```python
from build123d import *

# Parameters (mm, degrees)
F1_DEPTH = 346.075
F3_DEPTH = 31.751
F5_DEPTH = 38.1


with BuildPart() as f1:
    # F0 (on Front) → F1 (new body)
    with BuildSketch(Plane.XZ):
        with BuildLine():
            Line((0, -25.4), (0, 0))
            Line((0, 0), (25.4, 0))
            ThreePointArc((25.4, 0), (23.5401280605, 4.4901280605), (19.05, 6.35))
            Line((19.05, 6.35), (0, 6.35))
            ThreePointArc((0, 6.35), (-4.4901280605, 4.4901280605), (-6.35, 0))
            Line((-6.35, 0), (-6.35, -19.05))
            ThreePointArc((-6.35, -19.05), (-4.4901280605, -23.5401280605), (0, -25.4))
        make_face()
    extrude(amount=F1_DEPTH)

    # F2 (on face) → F3 (cut, through all)
    with BuildSketch(Plane.XY.offset(6.35)):
        Polygon((31.0680039475, -308.6569960525), (19.05, -320.675), (19.05, -346.075), (25.9507503361, -346.075), align=None)
        Polygon((19.05, -320.675), (0, -339.725), (0, -346.075), (19.05, -346.075), align=None)
        Polygon((0, -339.725), (-6.35, -346.075), (0, -346.075), align=None)
    extrude(amount=-F3_DEPTH, mode=Mode.SUBTRACT)

    # F4 (on face) → F5 (cut)
    with BuildSketch(Plane.XY.offset(6.35)):
        Polygon((25.4, 0), (-6.35, 0), (25.4, -31.75), align=None)
    extrude(amount=-F5_DEPTH, mode=Mode.SUBTRACT)


solid = f1.part
```
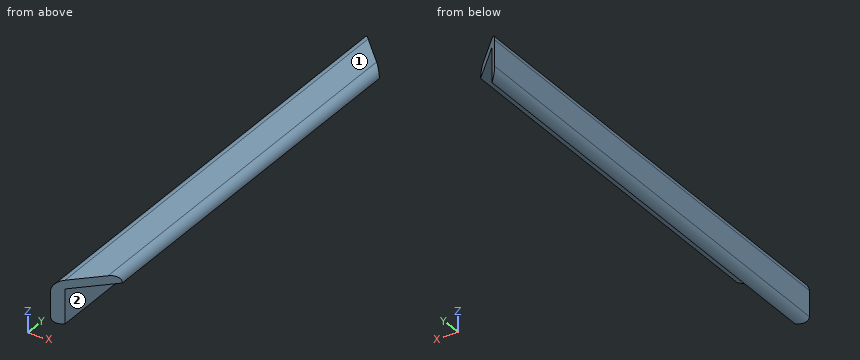
Work out the finished part from the listing and answer in its coordinate system (mm). Face numbers are marked on the shaded views. A direction names the side the tool comes from. Round coordinates to 2 decimals unless told otherwise and drop trailing zeros. Loops run counter-clockwise (first coordinate to the right, second up) from the corner with the lowest first, then second, coordinate; pieces in that order, holes last. Notation, with made-up numbers: (42.25, -33.5) -> (66.25, -33.5) arc R16 cw to (66.25, -19.5) -> close; hole circle Ø8 at (56, 73.25). An arc over 180 degrees is marked (long way). Write each question's results on one line, items separated by ' | '. Start each with the question number.
1. Given pin 1 Ø5 at (y, z) = (-50, -3) entering from +X; pin 2 Ø5 at (x, y) = (22, -143) entering from -Z; pin 3 Ø2 at (x, z) = (-3, -1) entering from +Y, each flat-ended and moving along its own axis, determine where each tip first touches the part or whether it passes through.
2. A tool of negligible diameter and unlimited length cuts with its end or side. For the marked faces 1 and 2, from which of +Z, -Z, +X, -X, +Y, -Y can it reach the whole face along a straight path? Write none if from no direction.
3. Section A-A (y = -167) is taken. Determine the outline of the cut face in (x, z), plus the area to 3 significant figures.
4. Section C-C (x = 9) is taken. Determine the outline of the cut face in (y, z) (3 decimals).
5. Find the intervals of material crossed by probe 1 along Z at (x, y) = (3.5, -52); probe 2 along X at (y, z) = (-286, -7), in increasing order. Write a range as from..to.
6. Section B-B (z = -12) is taken. Determine the outline of the cut face in (x, y) (3 decimals).
Evaluation:
1) pin 1: stops at x = 0 | pin 2: stops at z = 0 | pin 3: stops at y = -2.35
2) face 1: +Z, +X, -X, +Y, -Y | face 2: -Z, +X, +Y, -Y
3) outline: (-6.35, -19.05) arc R6.35 ccw to (0, -25.4) -> (0, 0) -> (25.4, 0) arc R6.35 ccw to (19.05, 6.35) -> (0, 6.35) arc R6.35 ccw to (-6.35, 0) -> close | area: 337 mm2
4) outline: (-330.725, 0) -> (-15.35, 0) -> (-15.35, 6.35) -> (-330.725, 6.35) -> close
5) probe 1: z = 0..6.35 | probe 2: x = -6.35..0
6) outline: (-6.35, -346.075) -> (0, -339.725) -> (0, -6.35) -> (-6.35, 0) -> close
